Can you work these out from the model? Positions are in its coordinate system, mm. A direction names the side the tool comes from. Give positions to 0.01 mm unless a question says otherwise; leave off trailing zeros. Order: outer loops, then holes, each group sorted by start corner. A loop starts at its lowest first (then second) coordinate and runs counter-clockwise, first axis right, second up. Notation, with made-up numbers: M 37.25,81 L 89.25,81 A7 cw 89.25,92 Z; hole C 1,2 d6. An arc over 180 degrees is marked long. One line per question, with ' | ' between items. Start each with the question number.
1) If we section it at D-D, the plane y = 74.5: Please give me the cut outline in (x, z).
2) I'm going to push flat-ended pins straight in: pin 1 Ø6 at (x, z) = (9.5, 85) entering from +Y; pin 2 Ø6 at (x, z) = (29.5, 86) entering from +Y; pin 3 Ø5.5 at (y, z) = (46.5, 91) entering from +X. Where does each tip first touch, or does it pass through?
3) Please list where these lines run through material, in increasing order: line 1 along X through (y, z) = (69, 81); line 2 along Y through (x, z) = (0, 89.75); line 3 along X through (y, z) = (29.5, 89). Write a range as [from, to].
4) If we section it at C-C, the plane z = 89.25: State how many separate pieces and enclosed holes the cut face has, plus the area to 3 significant figures.
5) Thinking about a two-plate mould opening in Y: for faces 4 (the flat face through (36.44, 31.75, 86)), 5 (the flat face through (-25.4, 51, 88)), 6 (the cylindrical face through (-2.36, 87.827, 88.119)), which applies, +Y half, -Y half, draft (parallel to the pull), parting line (faces both ways), or undercut?
6) For faces 1 (the flat face through (25.4, 51, 88)), 2 (the flat face through (-37, 31.75, 86)), 3 (the cylindrical face through (29.991, 24.058, 90.166)), which set-ups out of +Z, -Z, +X, -X, +Y, -Y let a thin tool reach every point of the face, with its end or its side?
7) If we section it at B-B, the plane y = 55.5: Please give me the cut outline in (x, z), plus the area to 3 significant figures.
8) If we section it at A-A, the plane z = 94.75: Please give me the cut outline in (x, y), plus the area to 3 significant figures.
```python
from build123d import *

# Parameters (mm, degrees)
SKETCH1_W                                         = 74.3632
SKETCH1_H                                         = 19.05
BOSS_EXTRUDE2_DEPTH                               = 76.2
SKETCH2_R                                         = 18.1316
CUT_EXTRUDE1_DEPTH                                = 20.05
CSK_FOR_8_FLAT_HEAD_MACHINE_SCREW_100_D           = 4.9149
CSK_FOR_8_FLAT_HEAD_MACHINE_SCREW_100_CSINK_D     = 10.9728
CSK_FOR_8_FLAT_HEAD_MACHINE_SCREW_100_CSINK_ANGLE = 100


with BuildPart() as part:
    # Sketch1 → Boss-Extrude2 (new body)
    with BuildSketch(Plane(origin=(0, 19.05, 0), x_dir=(1, 0, 0), z_dir=(0, 1, 0))):
        with Locations((0, -87.9856)):
            Rectangle(SKETCH1_W, SKETCH1_H)
    extrude(amount=BOSS_EXTRUDE2_DEPTH)

    # Sketch2 → Cut-Extrude1 (cut, through all)
    with BuildSketch(Plane.XY.offset(97.5106)):
        with BuildLine():
            Line((-37.1816, 95.25), (-37.1816, 31.75))
            Line((-37.1816, 31.75), (-25.4, 31.75))
            Line((-25.4, 31.75), (-25.4, 69.85))
            ThreePointArc((-25.4, 69.85), (-17.960512267, 87.810512217), (-7.1e-08, 95.25))
            Line((-7.1e-08, 95.25), (-37.1816, 95.25))
        make_face()
        with BuildLine():
            Line((25.4, 69.85), (25.4, 31.75))
            Line((25.4, 31.75), (37.1816, 31.75))
            Line((37.1816, 31.75), (37.1816, 95.25))
            Line((37.1816, 95.25), (-7.1e-08, 95.25))
            ThreePointArc((-7.1e-08, 95.25), (17.960512217, 87.810512267), (25.4, 69.85))
        make_face()
        with Locations((0, 69.85)):
            Circle(SKETCH2_R)
    extrude(amount=-CUT_EXTRUDE1_DEPTH, mode=Mode.SUBTRACT)

    # CSK for #8 Flat Head Machine Screw (100)1 (through all)
    with Locations(Plane(origin=(0, 31.75, 0), x_dir=(1, 0, 0), z_dir=(0, 1, 0))):
        with Locations((-31.125, -87.9856), (31.125, -87.9856)):
            CounterSinkHole(CSK_FOR_8_FLAT_HEAD_MACHINE_SCREW_100_D / 2, CSK_FOR_8_FLAT_HEAD_MACHINE_SCREW_100_CSINK_D / 2, counter_sink_angle=CSK_FOR_8_FLAT_HEAD_MACHINE_SCREW_100_CSINK_ANGLE)


solid = part.part
```
Results found:
1) outline: M -24.97,78.46 L -17.53,78.46 L -17.53,97.51 L -24.97,97.51 Z; M 17.53,78.46 L 24.97,78.46 L 24.97,97.51 L 17.53,97.51 Z
2) pin 1: stops at y = 94.4 | pin 2: stops at y = 31.75 | pin 3: stops at x = 25.4
3) line 1: x = [-25.4, -18.11], [18.11, 25.4] | line 2: y = [19.05, 51.72], [87.98, 95.25] | line 3: x = [-37.18, -33.74], [-28.51, 28.51], [33.74, 37.18]
4) separate pieces: 3 | enclosed holes: 1 | area: 2,740 mm²
5) face 4: +Y half | face 5: draft | face 6: undercut
6) face 1: +Z, -Z, +X, +Y | face 2: +Z, -Z, -X, +Y | face 3: +Y, -Y
7) outline: M -25.4,78.46 L -11.08,78.46 L -11.08,97.51 L -25.4,97.51 Z; M 11.08,78.46 L 25.4,78.46 L 25.4,97.51 L 11.08,97.51 Z | area: 545 mm²
8) outline: M -37.18,19.05 L 37.18,19.05 L 37.18,31.75 L 25.4,31.75 L 25.4,69.85 A25.4 ccw -25.4,69.85 L -25.4,31.75 L -37.18,31.75 Z; hole C 0,69.85 d36.26 | area: 2,860 mm²
